Source: CAD feature listing. Evaluate the final solid. Frame: model axes, mm. A direction names the side the tool comes from. Give positions to 0.01 mm unless a question says otherwise; leave off trailing zeros. Loops run counter-clockwise (first coordinate to the right, second up) from the corner with the lowest first, then second, coordinate; pieces in that order, holes last. Notation, with made-up numbers: (22.25, 83) -> (36.25, 83) arc R19 cw to (36.25, 106) -> close; hole circle Ø5 at (17.5, -2.75). An arc over 180 degrees is marked (long way). Return JSON: item names as keys, results as strings. Group by question number.
(1) Access query for faces 1 (the face through (112.998, 203.452, -26.922)), 2 (the face through (105, 195.484, -19)), 3 (the face through (114.605, 195, -19)). Directions: +Z, -Z, +X, -X, +Y, -Y. A direction counts if a zero-diameter tool reaches every point of the face in a straight line with its end or side. Return the directions, or none.
(2) Cut plane C-C on y = 208.75. Return loops of the section in (x, z), then the cut area to 3 significant figures.
(3) Cut plane D-D on x = 118.5. Return loops of the section in (y, z), then the cut area to 3 significant figures.
(4) Draft query along Y for faces 4 (the face through (101.606, 199, -19)), 5 (the face through (111.42, 212.82, -19.83)), 6 (the face through (112, 193.684, -19)). Return one class per face: released by +Y, released by -Y, zero draft, split by the parting line, or undercut.
(5) Cut plane B-B on x = 112. Return loops of the section in (y, z), then the cut area to 3 significant figures.
(6) Pin query (flat end, axial travel): pin 1 (11 mm diameter, centred on x = 111.56, z = -6.5, fed in from +Y); pin 2 (7.5 mm diameter, centred on x = 113.5, z = -33, fed in from +Y); pin 3 (5.5 mm diameter, centred on x = 111.56, z = -6.5, fed in from -Y); pin 4 (0.5 mm diameter, centred on y = 194.5, z = -25, fed in from -X). Return the tip coordinate at first contact, or that it passes through.
(7) Ray query, line 1 (X direction, y = 208, z = -28); line 2 (Y direction, x = 107, z = -15); line 3 (Z direction, x = 118, y = 201.75). Return the intervals inside material, ascending. Write a range as from..to.
(8) Cut plane A-A on z = -19. Return loops of the section in (x, y).
```python
from build123d import *

# Parameters (mm, degrees)
BOSS_EXTRUDE1_DEPTH = 38
SKETCH2_R           = 6.39
BOSS_EXTRUDE2_DEPTH = 19.9


with BuildPart() as part:
    # Sketch1 → Boss-Extrude1 (new body)
    with BuildSketch(Plane.XY):
        Polygon((101.60617691, 195.484265545), (108.51617691, 195.484265545), (108.51617691, 193.684265545), (114.604851948, 193.684265545), (114.604851948, 195.484265545), (121.50617691, 195.484265545), (121.50617691, 198.484265545), (101.60617691, 198.484265545), align=None)
    extrude(amount=-BOSS_EXTRUDE1_DEPTH)

    # Sketch2 → Boss-Extrude2 (add)
    with BuildSketch(Plane.ZY.offset(-101.60617691)):
        with BuildLine():
            Line((-38, 198.484265545), (-25.235062395, 212.261288734))
            ThreePointArc((-25.235062395, 212.261288734), (-19, 214.984265545), (-12.764937605, 212.261288734))
            Line((-12.764937605, 212.261288734), (0, 198.484265545))
            Line((0, 198.484265545), (-38, 198.484265545))
        make_face()
        with Locations((-19, 206.484265545)):
            Circle(SKETCH2_R, mode=Mode.SUBTRACT)
    extrude(amount=-BOSS_EXTRUDE2_DEPTH)

    # Sketch3 → Cut-Revolve1 (revolve, cut)
    with BuildSketch(Plane.ZY.offset(-111.55617691)):
        Polygon((-26.7, 211.670017018), (-26.7, 198.985665545), (-28.5, 198.985665545), (-28.5, 189.906068288), (-31.5, 189.906068288), (-31.5, 211.670017018), align=None)
    cut_revolve1 = revolve(axis=Axis((111.55617691, 189.906068288, -31.5), (0, 1, 0)), mode=Mode.SUBTRACT)

    # Mirror1: Cut-Revolve1 across plane
    add(cut_revolve1.mirror(Plane(origin=(0, 0, -19), x_dir=(1, 0, 0), z_dir=(0, 0, -1))), mode=Mode.SUBTRACT)


solid = part.part
```
Answers:
{
 "1": {"face 1": "+Y", "face 2": "+Z, -Z, -X, -Y", "face 3": "+Z, -Z, +X, -Y"},
 "2": {"outline": "(101.61, -28.49) -> (107.82, -28.49) arc R4.8 cw to (115.29, -28.49) -> (121.51, -28.49) -> (121.51, -24.97) -> (101.61, -24.97) -> close; (101.61, -13.03) -> (121.51, -13.03) -> (121.51, -9.51) -> (115.29, -9.51) arc R4.8 cw to (107.82, -9.51) -> (101.61, -9.51) -> close", "area": "121 mm²"},
 "3": {"outline": "(195.48, -38) -> (198.48, -38) -> (212.26, -25.24) arc R8.5 ccw to (212.26, -12.76) -> (198.48, 0) -> (195.48, 0) -> close; hole circle Ø12.78 at (206.48, -19)", "area": "357 mm²"},
 "4": {"face 4": "zero draft", "face 5": "undercut", "face 6": "released by -Y"},
 "5": {"outline": "(193.68, -38) -> (198.48, -38) -> (200.34, -36.28) -> (198.99, -36.28) -> (198.99, -34.47) -> (193.68, -34.47) -> close; (193.68, -28.53) -> (198.99, -28.53) -> (198.99, -26.72) -> (210.66, -26.72) -> (212.26, -25.24) arc R8.5 ccw to (212.26, -12.76) -> (210.66, -11.28) -> (198.99, -11.28) -> (198.99, -9.47) -> (193.68, -9.47) -> close; (193.68, -3.53) -> (198.99, -3.53) -> (198.99, -1.72) -> (200.34, -1.72) -> (198.48, 0) -> (193.68, 0) -> close; hole circle Ø12.78 at (206.48, -19)", "area": "238 mm²"},
 "6": {"pin 1": "y = 211.44", "pin 2": "y = 206.65", "pin 3": "through", "pin 4": "x = 108.52"},
 "7": {"line 1": "101.61..108.27, 114.84..121.51", "line 2": "195.48..201.5, 211.47..213.98", "line 3": "-34.97..-23.29, -14.71..-3.03"},
 "8": {"outline": "(101.61, 195.48) -> (108.52, 195.48) -> (108.52, 193.68) -> (114.6, 193.68) -> (114.6, 195.48) -> (121.51, 195.48) -> (121.51, 200.09) -> (101.61, 200.09) -> close; (101.61, 212.87) -> (121.51, 212.87) -> (121.51, 214.98) -> (101.61, 214.98) -> close"}
}
